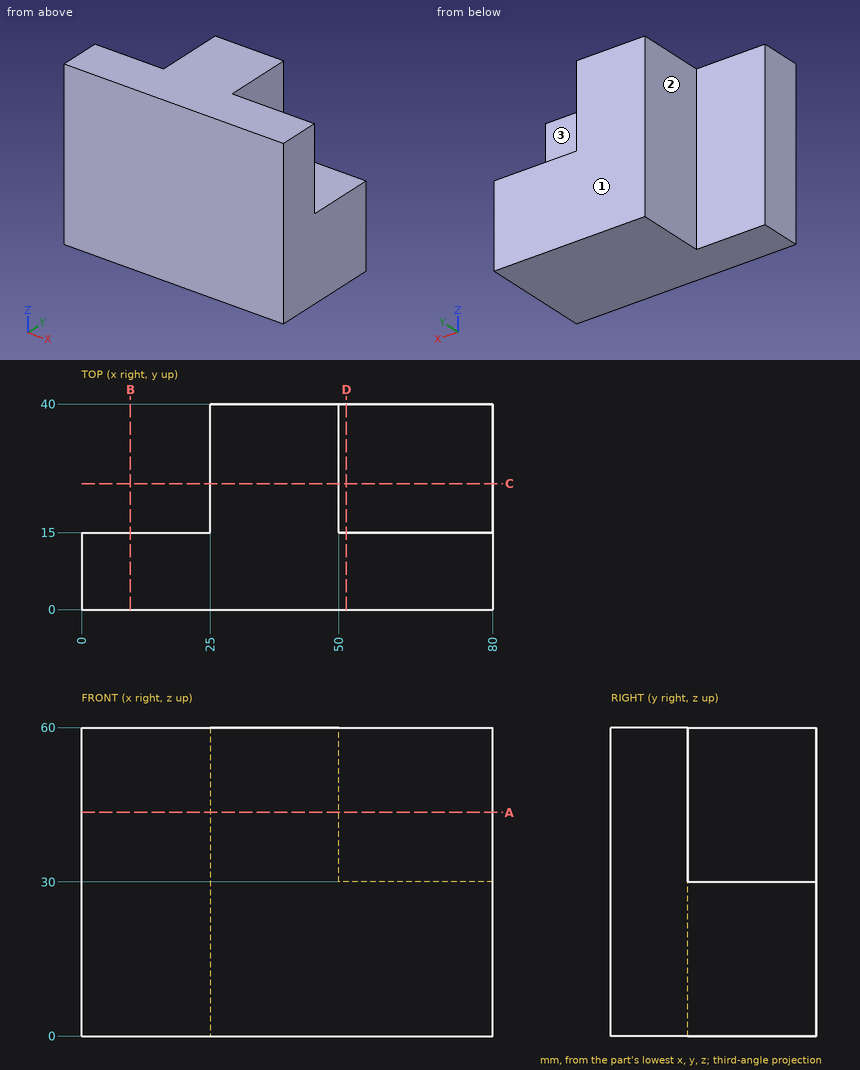
Job drawing, mm, ordinate dimensions from the low corner. One solid piece. A direction names the side the tool comes from. Give positions to 0.01 mm unless a question says otherwise; leave off trailing zeros. Order: outer loops, then holes, each group sorted by start corner. A loop starts at its lowest first (then second) coordinate and runs counter-clockwise, first axis right, second up. Notation, with made-up numbers: (-39, 75) - (-29, 75) arc R30 cw to (-29, 107) - close; hole circle Ø1 at (33.25, 66.5). An arc over 180 degrees is marked (long way). Return JSON: item names as keys, results as strings.
1) Flat gauge pins, fed straight in: P1, Ø8, axis at y = 34, z = 33.5, coming from the -X side; P2, Ø12.5, axis at x = 10, z = 31, coming from the +Y side; P3, Ø7.5, axis at y = 30.5, z = 42, coming from the +X side. Where does each tip first touch, or does it go through?
Geometry says:
{"P1": "x = 25", "P2": "y = 15", "P3": "x = 50"}
2) Cut at B-B, the plane x = 9.5. Give the cut face in (y, z).
Geometry says:
{"outline": "(0, 0) - (15, 0) - (15, 60) - (0, 60) - close"}
3) Probe line 1 (X direction, y = 33, z = 48); line 2 (Y direction, x = 13, z = 47); line 3 (X direction, y = 36.5, z = 12). List the from-to ranges inside material, lowest first. Write a range as from..to.
Geometry says:
{"line 1": "25..50", "line 2": "0..15", "line 3": "25..80"}
4) Cut at C-C, the plane y = 24.5. Give the cut face in (x, z).
Geometry says:
{"outline": "(25, 0) - (80, 0) - (80, 30) - (50, 30) - (50, 60) - (25, 60) - close"}
5) Cut at A-A, the plane z = 43.5. Give the cut face in (x, y), plus the area to 4 significant figures.
Geometry says:
{"outline": "(0, 0) - (80, 0) - (80, 15) - (50, 15) - (50, 40) - (25, 40) - (25, 15) - (0, 15) - close", "area": "1,825 mm²"}
6) Cut at D-D, the plane x = 51.5. Give the cut face in (y, z), plus the area to 3 significant figures.
Geometry says:
{"outline": "(0, 0) - (40, 0) - (40, 30) - (15, 30) - (15, 60) - (0, 60) - close", "area": "1,650 mm²"}
7) 3-axis set-ups, long thin cutter, end or side, ignore diameter. For the marked faces 1, 2 and 3: which of +Z, -Z, +X, -X, +Y, -Y reach the whole face in a straight line?
Geometry says:
{"face 1": "+Z, -Z, +X, -X, +Y", "face 2": "+Z, -Z, -X, +Y", "face 3": "+Z, +X, +Y"}
